Autodesk Inventor part; units mm, degrees
ref_plane "YZ Plane" through (0, 0, 0) normal (1, 0, 0) x (0, 1, 0)
ref_plane "XZ Plane" through (0, 0, 0) normal (0, 1, 0) x (-1, 0, 0)
ref_plane "XY Plane" through (0, 0, 0) normal (0, 0, 1) x (1, 0, 0)
sketch "Sketch1" plane through (0, 0, 0) normal (0, 0, 1) x (1, 0, 0)
  circle A0 centre (0, 0) radius 14
  dimension "d0" = 28
extrude "Extrusion1" add sketch "Sketch1" against normal blind 105
sketch "Sketch2" plane through (0, 0, 0) normal (0, 0, 1) x (1, 0, 0)
  circle A0 centre (0, 0) radius 14
  circle A1 centre (0, 0) radius 12
  dimension "d3" = 2
extrude "Extrusion2" add sketch "Sketch2" along normal blind 10 contours A1
sketch "Sketch3" plane through (0, 0, -105) normal (0, 0, -1) x (-1, 0, 0)
  circle A0 centre (0, 0) radius 12
extrude "Extrusion3" add sketch "Sketch3" along normal blind 10
fillet "Fillet1" radius 1 4 edges at (-12, 0, 0) (-14, 0, 0) (-14, 0, -105) (12, 0, -105)
sketch "Sketch4" plane through (0, 0, 10) normal (0, 0, 1) x (1, 0, 0)
  circle A0 centre (0, 0) radius 12
  circle A1 centre (0, 0) radius 9
  dimension "d9" = 3
extrude "Extrusion4" cut sketch "Sketch4" against normal through all contours A1
sketch "Sketch5" plane through (0, 0, 10) normal (0, 0, 1) x (1, 0, 0)
  line L0 (0, -18.4925) -> (0, 18.8644)
  line L1 (-0.55, -18.4925) -> (-0.55, 18.8644)
  line L2 (-0.55, -18.4925) -> (-0.55, -24.6298)
  line L3 (-0.55, -24.6298) -> (18.7736, -14.0631)
  line L4 (18.7736, -14.0631) -> (17.813, 9.6853)
  line L5 (17.813, 9.6853) -> (0, 24.9482)
  line L6 (0, 24.9482) -> (-0.55, 18.8644)
  point P0 (0, 0)
  dimension "d12" = 0.55
extrude "Extrusion5" cut sketch "Sketch5" against normal through all
properties part number "handle"
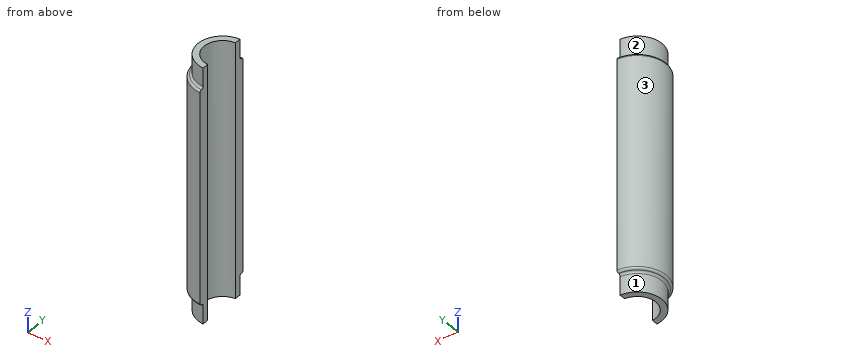
Geometry: final body of the model. Coordinates: model frame, mm. Face numbers are marked on the shaded views. A direction names the side the tool comes from. Give positions to 0.01 mm unless a question says otherwise; leave off trailing zeros. Answer as CSV lines item,"result". Start each with the question number.
1. Pin query (flat end, axial travel): P1, Ø5, axis at x = -5, y = 4, coming from the +Z side; P2, Ø2, axis at x = -5.5, z = -85.5, coming from the +Y side; P3, Ø1.5, axis at x = -2.5, z = -96.5, coming from the -Y side. Return the tip coordinate at first contact, or that it passes through.
2. Reachability of the marked faces 1, 2 and 3 from +Z, -Z, +X, -X, +Y, -Y: full face, straight path, thin tool, end or side. Return the list, or none.
3. Ray query, L1, parallel to Y at x = -2.5, z = -31; L2, parallel to Y at x = -2, z = -68; L3, parallel to Y at x = -10.75, z = -2. Return the intervals inside material, ascending.
Answers:
1,P1,"passes through"
1,P2,"stops at y = 13.26"
1,P3,"stops at y = -13.89"
2,face 1,"-Z, -X"
2,face 2,"+Z, -X"
2,face 3,"+Z, -Z, -X"
3,L1,"y = -13.77 to -8.65, 8.65 to 13.77"
3,L2,"y = -13.86 to -8.77, 8.77 to 13.86"
3,L3,"y = -8.97 to 8.97"
